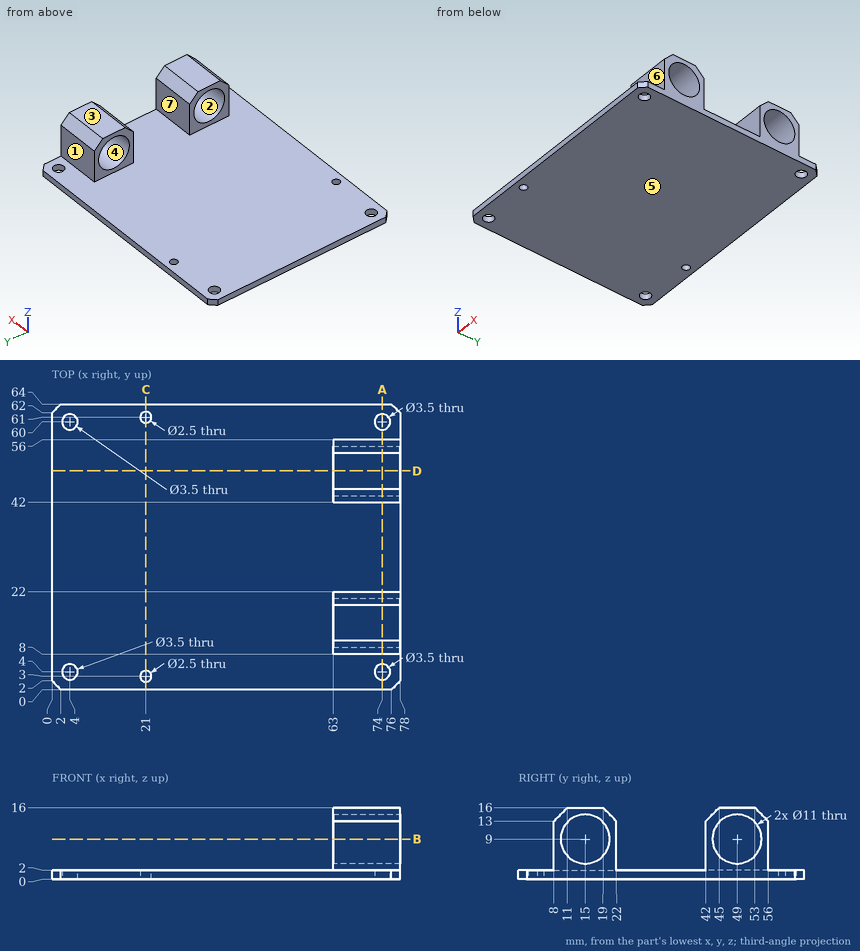
Study the drawing (mm; zero at the part's minimum x, y, z) and answer. A direction names the side the tool comes from. Round coordinates to 2 decimals unless told otherwise and drop trailing zeros. Loops run counter-clockwise (first coordinate to the right, second up) from the corner with the lowest first, then second, coordinate; pieces in that order, holes last.
Q1. For a pull along Y with two mould halves and no side action, classify the marked faces 1, 2, 3 and 4 as released by +Y, released by -Y, zero draft, split by the parting line, or undercut.
Q2. Given pin 1 Ø5 at (x, y) = (68.5, 48) entering from -Z; pin 2 Ø3.5 at (x, z) = (68.5, 9.5) entering from +Y; pin 3 Ø5.5 at (x, z) = (73.5, 5.5) entering from -Y; pin 4 Ø4 at (y, z) = (13, 6) entering from -X, each flat-ended and moving along its own axis, determine where each tip first touches the part or whether it passes through.
Q3. Find the intervals of material crossed by line 1 (Y direction, x = 74, z = 0.9); line 2 (Y direction, x = 21, z = 0.4); line 3 (Z direction, x = 68.5, y = 61.5), in increasing order.
Q4. Section D-D, the plane y = 49 is taken. Determine the outline of the cut face in (x, z), then the cut area to 3 significant figures.
Q5. Section B-B, the plane z = 9 is taken. Determine the outline of the cut face in (x, y).
Q6. Section C-C, the plane x = 21 is taken. Determine the outline of the cut face in (y, z).
Q7. Which of the six approach directions +Z, -Z, +X, -X, +Y, -Y give full straight-line access (tool end or side, diameter ignored) to the marked faces 5, 6 and 7?
Q8. Section A-A, the plane x = 74 is taken. Determine the outline of the cut face in (y, z), then the cut area to 3 significant figures.
Completed:
1. face 1: released by +Y
1. face 2: undercut
1. face 3: zero draft
1. face 4: undercut
2. pin 1: stops at z = 0
2. pin 2: stops at y = 56
2. pin 3: stops at y = 8
2. pin 4: stops at x = 63
3. line 1: y = 0 to 2.25, 5.75 to 58.25, 61.75 to 64
3. line 2: y = 0 to 1.75, 4.25 to 59.75, 62.25 to 64
3. line 3: z = 0 to 2
4. outline: (0, 0) - (78, 0) - (78, 3.5) - (63, 3.5) - (63, 2) - (0, 2) - close; (63, 14.5) - (78, 14.5) - (78, 16) - (63, 16) - close
4. area: 201 mm2
5. outline: (63, 8) - (78, 8) - (78, 9.5) - (63, 9.5) - close; (63, 20.5) - (78, 20.5) - (78, 22) - (63, 22) - close; (63, 42) - (78, 42) - (78, 43.5) - (63, 43.5) - close; (63, 54.5) - (78, 54.5) - (78, 56) - (63, 56) - close
6. outline: (0, 0) - (1.75, 0) - (1.75, 2) - (0, 2) - close; (4.25, 0) - (59.75, 0) - (59.75, 2) - (4.25, 2) - close; (62.25, 0) - (64, 0) - (64, 2) - (62.25, 2) - close
7. face 5: -Z, +X, -X, +Y, -Y
7. face 6: +Z, +X, -X, -Y
7. face 7: +Z, +X, -X
8. outline: (0, 0) - (2.25, 0) - (2.25, 2) - (0, 2) - close; (5.75, 0) - (58.25, 0) - (58.25, 2) - (56, 2) - (56, 13) - (53, 16) - (45, 16) - (42, 13) - (42, 2) - (22, 2) - (22, 13) - (19, 16) - (11, 16) - (8, 13) - (8, 2) - (5.75, 2) - close; (61.75, 0) - (64, 0) - (64, 2) - (61.75, 2) - close; hole circle Ø11 at (15, 9); hole circle Ø11 at (49, 9)
8. area: 298 mm2
